from build123d import *

# Parameters (mm, degrees)
SKETCH1_R            = 88.9
SKETCH1_R_2          = 11.43
SKETCH1_R_3          = 2.159
SKETCH1_R_4          = 6.35
BODY_DEPTH           = 6.35
MOUNTING_TEETH_REACH = 127.884
SKETCH2_W            = 28.333333333
SKETCH2_H            = 6.35


with BuildPart() as part:
    # Sketch1 → Body (new body)
    with BuildSketch(Plane(origin=(0, 0, 0), x_dir=(1, 0, 0), z_dir=(0, 1, 0))):
        with Locations(Location((0, 0, 0), (0, 0, 270))):
            Circle(SKETCH1_R)
        with Locations(Location((0, 0, 0), (0, 0, 270))):
            Circle(SKETCH1_R_2, mode=Mode.SUBTRACT)
        with Locations(Location((0, 31.089, 0), (0, 0, 270))):
            Circle(SKETCH1_R_3, mode=Mode.SUBTRACT)
        with Locations(Location((26.923863778, -15.5445, 0), (0, 0, 270))):
            Circle(SKETCH1_R_3, mode=Mode.SUBTRACT)
        with Locations(Location((-26.923863778, -15.5445, 0), (0, 0, 270))):
            Circle(SKETCH1_R_3, mode=Mode.SUBTRACT)
        with Locations(Location((-18.648117099, 26.632271264, 0), (0, 0, 270))):
            Circle(SKETCH1_R_4, mode=Mode.SUBTRACT)
    extrude(amount=BODY_DEPTH)

    # Sketch2 → Mounting teeth (cut, up to next)
    with BuildSketch(Plane(origin=(0, 6.35, 0), x_dir=(1, 0, 0), z_dir=(0, 1, 0)), mode=Mode.PRIVATE) as mounting_teeth_sk1:
        with Locations((-28.333333334, 38.175)):
            Rectangle(SKETCH2_W, SKETCH2_H)
    mounting_teeth_tool1 = extrude(mounting_teeth_sk1.sketch, amount=-MOUNTING_TEETH_REACH, mode=Mode.PRIVATE) & part.part
    # Sketch2 → Mounting teeth (cut, up to next)
    with BuildSketch(Plane(origin=(0, 6.35, 0), x_dir=(1, 0, 0), z_dir=(0, 1, 0)), mode=Mode.PRIVATE) as mounting_teeth_sk2:
        with Locations((28.333333334, 38.175)):
            Rectangle(SKETCH2_W, SKETCH2_H)
    mounting_teeth_tool2 = extrude(mounting_teeth_sk2.sketch, amount=-MOUNTING_TEETH_REACH, mode=Mode.PRIVATE) & part.part
    # Sketch2 → Mounting teeth (cut, up to next)
    with BuildSketch(Plane(origin=(0, 6.35, 0), x_dir=(1, 0, 0), z_dir=(0, 1, 0)), mode=Mode.PRIVATE) as mounting_teeth_sk3:
        with Locations((28.333333334, -38.175)):
            Rectangle(SKETCH2_W, SKETCH2_H)
    mounting_teeth_tool3 = extrude(mounting_teeth_sk3.sketch, amount=-MOUNTING_TEETH_REACH, mode=Mode.PRIVATE) & part.part
    # Sketch2 → Mounting teeth (cut, up to next)
    with BuildSketch(Plane(origin=(0, 6.35, 0), x_dir=(1, 0, 0), z_dir=(0, 1, 0)), mode=Mode.PRIVATE) as mounting_teeth_sk4:
        with Locations((-28.333333334, -38.175)):
            Rectangle(SKETCH2_W, SKETCH2_H)
    mounting_teeth_tool4 = extrude(mounting_teeth_sk4.sketch, amount=-MOUNTING_TEETH_REACH, mode=Mode.PRIVATE) & part.part
    add(mounting_teeth_tool1.solids().sort_by_distance((-28.333333, 6.35, -38.175))[0], mode=Mode.SUBTRACT)
    add(mounting_teeth_tool2.solids().sort_by_distance((28.333333, 6.35, -38.175))[0], mode=Mode.SUBTRACT)
    add(mounting_teeth_tool3.solids().sort_by_distance((28.333333, 6.35, 38.175))[0], mode=Mode.SUBTRACT)
    add(mounting_teeth_tool4.solids().sort_by_distance((-28.333333, 6.35, 38.175))[0], mode=Mode.SUBTRACT)


solid = part.part
Geometry check sheet. Reference: the model listing, model coordinates, mm. Give positions to 0.01 mm unless a question says otherwise; leave off trailing zeros. Order: outer loops, then holes, each group sorted by start corner. A loop starts at its lowest first (then second) coordinate and runs counter-clockwise, first axis right, second up.
1) Draft check along X on faces 1 (the flat face through (-29, 3, -41.35)), 2 (the flat face through (1, 6.35, 19)), 3 (the cylindrical face through (74.96, 3.13, 47.79)). Enter one of: released by +X, released by -X, zero draft, split by the parting line, or undercut.
Results are:
face 1: undercut
face 2: zero draft
face 3: split by the parting line
2) Cross-section at C-C (y = 2.25). Give the number of separate pieces and of enclosed holes in the cut face, then the cut area to 3 significant figures.
Results are:
separate pieces: 1
enclosed holes: 9
area: 23,500 mm2
3) Material ranges on probe 1 along X at (y, z) = (2.5, 0); probe 2 along X at (y, z) = (3.75, 14.5); probe 3 along Z at (x, y) = (22, 5), recorded low to high.
Results are:
probe 1: x = -88.9 to -11.43, 11.43 to 88.9
probe 2: x = -87.71 to -28.81, -25.03 to 25.03, 28.81 to 87.71
probe 3: z = -86.13 to -41.35, -35 to 35, 41.35 to 86.13
4) Cross-section at D-D (x = -54.5). Record the boundary of the cut face in (y, z).
Results are:
outline: (0, -70.24) - (6.35, -70.24) - (6.35, 70.24) - (0, 70.24) - close
5) Cross-section at A-A (x = 0). Record the boundary of the cut face in (y, z), then the cut area to 3 significant figures.
Results are:
outline: (0, -88.9) - (6.35, -88.9) - (6.35, -33.25) - (0, -33.25) - close; (0, -28.93) - (6.35, -28.93) - (6.35, -11.43) - (0, -11.43) - close; (0, 11.43) - (6.35, 11.43) - (6.35, 88.9) - (0, 88.9) - close
area: 956 mm2
6) Cross-section at B-B (z = 0). Record the boundary of the cut face in (x, y).
Results are:
outline: (-88.9, 0) - (-11.43, 0) - (-11.43, 6.35) - (-88.9, 6.35) - close; (11.43, 0) - (88.9, 0) - (88.9, 6.35) - (11.43, 6.35) - close
7) Gauge pin test, flat ends, axial feed: pin 1 (3 mm diameter, centred on x = -18, y = 2.5, fed in from +Z); pin 2 (1 mm diameter, centred on x = 18.5, y = 0.5, fed in from +Z); pin 3 (3 mm diameter, centred on x = 2.5, y = 3, fed in from +Z); pin 4 (3.5 mm diameter, centred on x = 26.92, z = 15.54, fed in from +Y). Record the tip position at first contact, or that the pin passes through.
Results are:
pin 1: stops at z = 87.36
pin 2: stops at z = 87.06
pin 3: stops at z = 88.89
pin 4: passes through
